Verification items for the finished model (mm, model axes). Face numbers are marked on the shaded views. A direction names the side the tool comes from. Coordinates: 2 decimals unless noted, no trailing zeros. Order: outer loops, then holes, each group sorted by start corner. A loop starts at its lowest first (then second) coordinate and runs counter-clockwise, first axis right, second up. Notation, with made-up numbers: (30.5, 2.5) -> (75.5, 2.5) arc R23 cw to (75.5, 19.5) -> close; hole circle Ø10 at (7, 57.25). An arc over 180 degrees is marked (long way). Use CSV: the item, a comma, the result in double quotes. Start each with the question number.
1) Go/stop test with flat-tipped pins: pin 1 (18.5 mm diameter, centred on x = 0, z = 0, fed in from +Y); pin 2 (5 mm diameter, centred on x = -0.5, z = -0.5, fed in from +Y). Record where each tip stops, or that it passes through.
2) Sectioned sample at C-C on z = -0.5. Record the boundary of the cut face in (x, y), then the cut area to 3 significant figures.
3) Tool access check on the marked faces 1 and 2. Record the directions out of +Z, -Z, +X, -X, +Y, -Y that give a thin tool (end or side, any length) a straight path to the whole face; none if there is none.
4) Scan lines: line 1 along Z through (x, y) = (15, -6.5); line 2 along Z through (x, y) = (0, -9.1). Record each from-to range of solid material in increasing order.
5) Release check for a two-part mould opening along Z. For the marked faces 3, 4 and 5 record: released by +Z, released by -Z, zero draft, split by the parting line, or undercut.
6) Sectioned sample at A-A on x = 0. Record the boundary of the cut face in (y, z), then the cut area to 3 significant figures.
7) Sectioned sample at D-D on x = -9. Record the boundary of the cut face in (y, z).
8) Sectioned sample at B-B on y = -4.25. Record the boundary of the cut face in (x, z), then the cut area to 3 significant figures.
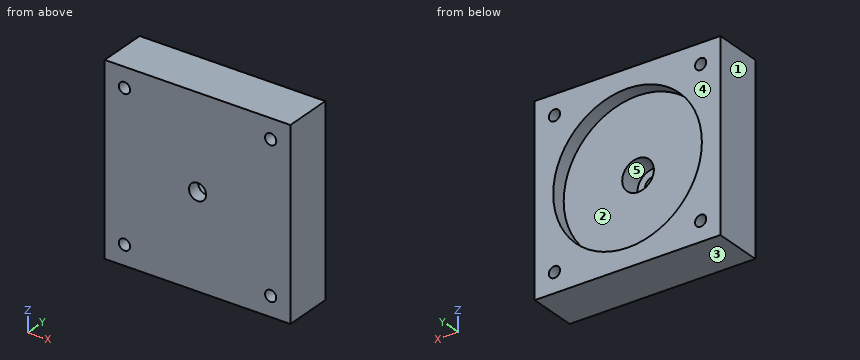
from build123d import *

# Parameters (mm, degrees)
SKETCH1_W           = 38.1
SKETCH1_H           = 38.1
BOSS_EXTRUDE1_DEPTH = 10
SKETCH1_3_R         = 1.15
CUT_EXTRUDE1_DEPTH  = 10
SKETCH1_4_R         = 1.15
CUT_EXTRUDE2_DEPTH  = 10
SKETCH1_5_R         = 1.15
CUT_EXTRUDE3_DEPTH  = 10
SKETCH1_6_R         = 1.15
CUT_EXTRUDE4_DEPTH  = 10
SKETCH1_7_R         = 15.25
SKETCH1_7_R_2       = 3.25
CUT_EXTRUDE5_DEPTH  = 3
SKETCH1_8_R         = 3.25
SKETCH1_8_R_2       = 1.75
CUT_EXTRUDE6_DEPTH  = 7.4
SKETCH1_9_R         = 1.75
CUT_EXTRUDE7_DEPTH  = 10


with BuildPart() as part:
    # Sketch1 → Boss-Extrude1 (new body)
    with BuildSketch(Plane(origin=(0, 0, 0), x_dir=(1, 0, 0), z_dir=(0, 1, 0))):
        Rectangle(SKETCH1_W, SKETCH1_H)
    extrude(amount=-BOSS_EXTRUDE1_DEPTH)

    # Sketch1<3> → Cut-Extrude1 (cut)
    with BuildSketch(Plane(origin=(0, 0, 0), x_dir=(1, 0, 0), z_dir=(0, 1, 0))):
        with Locations((-15, 15)):
            Circle(SKETCH1_3_R)
    extrude(amount=-CUT_EXTRUDE1_DEPTH, mode=Mode.SUBTRACT)

    # Sketch1<4> → Cut-Extrude2 (cut)
    with BuildSketch(Plane(origin=(0, 0, 0), x_dir=(1, 0, 0), z_dir=(0, 1, 0))):
        with Locations((15, 15)):
            Circle(SKETCH1_4_R)
    extrude(amount=-CUT_EXTRUDE2_DEPTH, mode=Mode.SUBTRACT)

    # Sketch1<5> → Cut-Extrude3 (cut)
    with BuildSketch(Plane(origin=(0, 0, 0), x_dir=(1, 0, 0), z_dir=(0, 1, 0))):
        with Locations((-15, -15)):
            Circle(SKETCH1_5_R)
    extrude(amount=-CUT_EXTRUDE3_DEPTH, mode=Mode.SUBTRACT)

    # Sketch1<6> → Cut-Extrude4 (cut)
    with BuildSketch(Plane(origin=(0, 0, 0), x_dir=(1, 0, 0), z_dir=(0, 1, 0))):
        with Locations((15, -15)):
            Circle(SKETCH1_6_R)
    extrude(amount=-CUT_EXTRUDE4_DEPTH, mode=Mode.SUBTRACT)

    # Sketch1<7> → Cut-Extrude5 (cut)
    with BuildSketch(Plane(origin=(0, 0, 0), x_dir=(1, 0, 0), z_dir=(0, 1, 0))):
        Circle(SKETCH1_7_R)
        Circle(SKETCH1_7_R_2, mode=Mode.SUBTRACT)
    extrude(amount=-CUT_EXTRUDE5_DEPTH, mode=Mode.SUBTRACT)

    # Sketch1<8> → Cut-Extrude6 (cut)
    with BuildSketch(Plane(origin=(0, 0, 0), x_dir=(1, 0, 0), z_dir=(0, 1, 0))):
        Circle(SKETCH1_8_R)
        Circle(SKETCH1_8_R_2, mode=Mode.SUBTRACT)
    extrude(amount=-CUT_EXTRUDE6_DEPTH, mode=Mode.SUBTRACT)

    # Sketch1<9> → Cut-Extrude7 (cut)
    with BuildSketch(Plane(origin=(0, 0, 0), x_dir=(1, 0, 0), z_dir=(0, 1, 0))):
        Circle(SKETCH1_9_R)
    extrude(amount=-CUT_EXTRUDE7_DEPTH, mode=Mode.SUBTRACT)


solid = part.part
Answers follow:
1,pin 1,"stops at y = -3"
1,pin 2,"stops at y = -7.4"
2,outline,"(-19.05, -10) -> (-1.68, -10) -> (-1.68, -7.4) -> (-3.21, -7.4) -> (-3.21, -3) -> (-15.24, -3) -> (-15.24, 0) -> (-19.05, 0) -> close; (1.68, -10) -> (19.05, -10) -> (19.05, 0) -> (15.24, 0) -> (15.24, -3) -> (3.21, -3) -> (3.21, -7.4) -> (1.68, -7.4) -> close"
2,area,"253 mm²"
3,face 1,"+Z, -Z, -X, +Y, -Y"
3,face 2,"+Y"
4,line 1,"z = -19.05 to -16.15, -13.85 to 13.85, 16.15 to 19.05"
4,line 2,"z = -19.05 to -1.75, 1.75 to 19.05"
5,face 3,"released by -Z"
5,face 4,"zero draft"
5,face 5,"undercut"
6,outline,"(-10, -19.05) -> (0, -19.05) -> (0, -15.25) -> (-3, -15.25) -> (-3, -3.25) -> (-7.4, -3.25) -> (-7.4, -1.75) -> (-10, -1.75) -> close; (-10, 1.75) -> (-7.4, 1.75) -> (-7.4, 3.25) -> (-3, 3.25) -> (-3, 15.25) -> (0, 15.25) -> (0, 19.05) -> (-10, 19.05) -> close"
6,area,"252 mm²"
7,outline,"(-10, -19.05) -> (0, -19.05) -> (0, -12.31) -> (-3, -12.31) -> (-3, 12.31) -> (0, 12.31) -> (0, 19.05) -> (-10, 19.05) -> close"
8,outline,"(-19.05, -19.05) -> (19.05, -19.05) -> (19.05, 19.05) -> (-19.05, 19.05) -> close; hole circle Ø2.3 at (-15, -15); hole circle Ø2.3 at (-15, 15); hole circle Ø6.5 at (0, 0); hole circle Ø2.3 at (15, -15); hole circle Ø2.3 at (15, 15)"
8,area,"1,400 mm²"
